```python
from build123d import *

# Parameters (mm, degrees)
F0_W     = 1193.8
F0_H     = 254
F1_DEPTH = 19.05
F2_W     = 19.05
F2_H     = 9.525
F3_DEPTH = 234.95
F4_W     = 1193.8
F4_H     = 6.35
F5_DEPTH = 9.525
F6_W     = 9.525
F6_H     = 19.05
F7_DEPTH = 25.4


with BuildPart() as f1:
    # F0 (on Top) → F1 (new body)
    with BuildSketch(Plane.XY):
        with Locations((596.9, 127)):
            Rectangle(F0_W, F0_H)
    extrude(amount=F1_DEPTH)

    # F2 (on face) → F3 (cut)
    with BuildSketch(Plane(origin=(0, 254, 0), x_dir=(-1, 0, 0), z_dir=(0, 1, 0))):
        with Locations((-298.45, 14.2875)):
            Rectangle(F2_W, F2_H)
        with Locations((-596.9, 14.2875)):
            Rectangle(F2_W, F2_H)
        with Locations((-895.35, 14.2875)):
            Rectangle(F2_W, F2_H)
    extrude(amount=-F3_DEPTH, mode=Mode.SUBTRACT)

    # F4 (on face) → F5 (cut)
    with BuildSketch(Plane.XY.offset(19.05)):
        with Locations((596.9, 250.825)):
            Rectangle(F4_W, F4_H)
    extrude(amount=-F5_DEPTH, mode=Mode.SUBTRACT)

    # F6 (on face) → F7 (cut)
    with BuildSketch(Plane.XY.offset(19.05)):
        with Locations((4.7625, 9.525)):
            Rectangle(F6_W, F6_H)
        with Locations((1189.0375, 9.525)):
            Rectangle(F6_W, F6_H)
    extrude(amount=-F7_DEPTH, mode=Mode.SUBTRACT)


solid = f1.part
```
Could you check a few things on this model? Use its own coordinates, in mm. A direction names the side the tool comes from. Give positions to 0.01 mm unless a question says otherwise; leave off trailing zeros. Loops run counter-clockwise (first coordinate to the right, second up) from the corner with the lowest first, then second, coordinate; pieces in that order, holes last. Notation, with made-up numbers: (-28.75, -8) - (17.25, -8) arc R8 cw to (17.25, 2) - close; hole circle Ø11 at (8, 80). An arc over 180 degrees is marked (long way). Use one line per item in the form item = value.
1. Thinking about a two-plate mould opening in X: for faces 1 (the face through (1184.275, 9, 10)), 2 (the face through (683, 250, 9.525)), 3 (the face through (589, 0, 9)), which applies, released by +X, released by -X, zero draft, split by the parting line, or undercut?
Response values:
face_1 = released by +X
face_2 = undercut
face_3 = zero draft
2. I'm going to push flat-ended pins straight in: pin 1 Ø5 at (x, z) = (298, 15) entering from +Y; pin 2 Ø2 at (x, y) = (296.5, 138.5) entering from +Z (3 decimals); pin 3 Ø5.5 at (y, z) = (6, 12) entering from +X (3 decimals); pin 4 Ø10.5 at (y, z) = (125.5, 12.5) entering from -X. Where does each tip first touch, or does it pass through?
Response values:
pin_1 = 19.05
pin_2 = 9.525
pin_3 = 1184.275
pin_4 = 0
3. On a 3-axis mill with a long thin cutter (end or side, diameter ignored), from which of +Z, -Z, +X, -X, +Y, -Y can I reach the whole of each face in a straight line? I mean faces 4 (the face through (1193.8, 135, 9)), 5 (the face through (9.525, 9, 10)). Say none if no direction works.
Response values:
face_4 = +Z, -Z, +X, +Y, -Y
face_5 = +Z, -Z, -X, -Y
4. I want a section at B-B (z = 15). Please give me the cut outline in (x, y) (3 decimals).
Response values:
outline = (0, 19.05) - (9.525, 19.05) - (9.525, 0) - (1184.275, 0) - (1184.275, 19.05) - (1193.8, 19.05) - (1193.8, 247.65) - (904.875, 247.65) - (904.875, 19.05) - (885.825, 19.05) - (885.825, 247.65) - (606.425, 247.65) - (606.425, 19.05) - (587.375, 19.05) - (587.375, 247.65) - (307.975, 247.65) - (307.975, 19.05) - (288.925, 19.05) - (288.925, 247.65) - (0, 247.65) - close
5. I need wall thicknesses on probe 1 along X at (y, z) = (109, 15.25) (3 decimals); probe 2 along Y at (x, z) = (261, 15.5); probe 3 along Z at (x, y) = (292.5, 83) (3 decimals). Which ranges of each line are inside material? Lowest first, please.
Response values:
probe_1 = 0 to 288.925, 307.975 to 587.375, 606.425 to 885.825, 904.875 to 1193.8
probe_2 = 0 to 247.65
probe_3 = 0 to 9.525
6. I want a section at A-A (y = 60). Please give me the cut outline in (x, z) (3 decimals).
Response values:
outline = (0, 0) - (1193.8, 0) - (1193.8, 19.05) - (904.875, 19.05) - (904.875, 9.525) - (885.825, 9.525) - (885.825, 19.05) - (606.425, 19.05) - (606.425, 9.525) - (587.375, 9.525) - (587.375, 19.05) - (307.975, 19.05) - (307.975, 9.525) - (288.925, 9.525) - (288.925, 19.05) - (0, 19.05) - close
